Read the model definition and answer for the solid it produces. Units are mm, in the model's axes. Give positions to 0.01 mm unless a question says otherwise; leave off trailing zeros. Order: outer loops, then holes, each group sorted by start corner. A loop starts at its lowest first (then second) coordinate and runs counter-clockwise, first axis right, second up. Notation, with made-up numbers: (39, 22) - (48, 22) arc R14 cw to (48, 44) - close; hole circle Ø4 at (27, 34). An arc over 180 degrees is marked (long way). Use a Markdown table: item, result. Add a question column.
1. A cutting plane is placed at B-B on z = 4. Determine the outline of the cut face in (x, y), and give its area (3 significant figures).
2. Consider L1, parallel to X at y = 536, z = 1.25; L2, parallel to Z at x = -4, y = 530.5; L3, parallel to X at y = 272.5, z = -5. Determine where each line is inside the solid, lowest interval first.
3. A cutting plane is placed at A-A on y = 522.5. Determine the outline of the cut face in (x, z), and give its area (3 significant figures).
Autodesk Inventor part; units mm, degrees
ref_plane "YZ Plane" through (0, 0, 0) normal (1, 0, 0) x (0, 1, 0)
ref_plane "XZ Plane" through (0, 0, 0) normal (0, 1, 0) x (-1, 0, 0)
ref_plane "XY Plane" through (0, 0, 0) normal (0, 0, 1) x (1, 0, 0)
sketch "Sketch1" plane through (0, 0, 0) normal (0, 1, 0) x (-1, 0, 0)
  line L0 (-3.6687, -6.3544) -> (-7.3374, 0)
  line L1 (-7.3374, 0) -> (-3.6687, 6.3544)
  line L2 (-3.6687, 6.3544) -> (3.6687, 6.3544)
  line L3 (3.6687, 6.3544) -> (7.3374, 0)
  line L4 (7.3374, 0) -> (3.6687, -6.3544)
  line L5 (3.6687, -6.3544) -> (-3.6687, -6.3544)
  point P0 (0, 0)
  point P1 (0, 0)
extrude "Extrusion1" add sketch "Sketch1" along normal blind 591.4136
properties part number "Elevator Drive Shaft"
Output values:
| question | item | result |
|---|---|---|
| 1 | outline | (-5.03, 0) - (5.03, 0) - (5.03, 591.41) - (-5.03, 591.41) - close |
| 1 | area | 5,950 mm² |
| 2 | L1 | -6.62 to 6.62 |
| 2 | L2 | -5.78 to 5.78 |
| 2 | L3 | -4.45 to 4.45 |
| 3 | outline | (-7.34, 0) - (-3.67, -6.35) - (3.67, -6.35) - (7.34, 0) - (3.67, 6.35) - (-3.67, 6.35) - close |
| 3 | area | 140 mm² |
